from build123d import *

# Parameters (mm, degrees)
SKETCH1_R           = 76.2
BOSS_EXTRUDE1_DEPTH = 130
SKETCH1_3_R         = 72.2
CUT_EXTRUDE1_DEPTH  = 126
FILLET1_R           = 5


with BuildPart() as part:
    # Sketch1 → Boss-Extrude1 (new body)
    with BuildSketch(Plane(origin=(0, 0, 0), x_dir=(1, 0, 0), z_dir=(0, 1, 0))):
        with Locations(Location((0, 0, 0), (0, 0, 270))):
            Circle(SKETCH1_R)
        with BuildLine():
            Line((-3.175, -5), (-3.175, 5))
            ThreePointArc((-3.175, 5), (0, 8.175), (3.175, 5))
            Line((3.175, 5), (3.175, -5))
            ThreePointArc((3.175, -5), (0, -8.175), (-3.175, -5))
        make_face(mode=Mode.SUBTRACT)
    extrude(amount=BOSS_EXTRUDE1_DEPTH)

    # Sketch1<3> → Cut-Extrude1 (cut)
    with BuildSketch(Plane(origin=(0, 0, 0), x_dir=(1, 0, 0), z_dir=(0, 1, 0))):
        with Locations(Location((0, 0, 0), (0, 0, 270))):
            Circle(SKETCH1_3_R)
    extrude(amount=CUT_EXTRUDE1_DEPTH, mode=Mode.SUBTRACT)

    # Fillet1
    fillet1_edges = [part.edges().sort_by_distance(p)[0] for p in [
        (0, 130, -76.2),
    ]]
    fillet(fillet1_edges, radius=FILLET1_R)


solid = part.part
The model under review builds one solid part; all positions refer to its coordinate system, in mm. A direction names the side the tool comes from. Give positions to 0.01 mm unless a question says otherwise; leave off trailing zeros. Write each loop counter-clockwise with the first axis right and the second up, starting at its lowest first coordinate (ties: lowest second). Pieces come first, ordered by that corner, then holes.
1. For P1, Ø6, axis at x = 23, z = -51.5, coming from the -Y side; P2, Ø10, axis at y = 16.5, z = -9, coming from the -X side; P3, Ø8, axis at y = 60.5, z = 44.5, coming from the -X side, all flat-tipped, find the tip position at first contact; note any pin that passes through.
2. Tool access review of faces 1 (the flat face through (-15, 130, -1)), 2 (the flat face through (-3.175, 128, 0)), 3 (the cylindrical face through (-43.933, 62.118, -57.295)): name each direction out of +Z, -Z, +X, -X, +Y, -Y from which nothing blocks a thin tool from reaching the whole face with its end or side.
3. Add section B-B, the plane x = 0. Write out the cut boundary in (y, z) (3 decimals), plus the area to 3 significant figures.
4. Wall thickness on L1, parallel to X at y = 67, z = 0; L2, parallel to Z at x = 21.5, y = 71.5; L3, parallel to Y at x = 25, z = -61.5: over which ranges is each line inside the solid? List them lowest first.
5. Add section C-C, the plane y = 27.5. Write out the cut boundary in (x, z).
6. Draft analysis for pull direction X (two halves, no side actions). For faces 4 (the cylindrical face through (-46.367, 61.625, -60.47)), 5 (the flat face through (46, 0, 56)), 6 (the cylindrical face through (-0.07, 127.972, -8.174)), state which applies: +X half, -X half, draft (parallel to the pull), parting line (faces both ways), or undercut.
7. Add section A-A, the plane z = 0. Write out the cut boundary in (x, y) (3 decimals).
Worked answers:
1. P1: stops at y = 126
1. P2: stops at x = -76.09
1. P3: stops at x = -64.55
2. face 1: +Z, -Z, +X, -X, +Y
2. face 2: +Y, -Y
2. face 3: -Y
3. outline: (0, -76.2) - (125, -76.2) arc R5 ccw to (130, -71.2) - (130, -8.175) - (126, -8.175) - (126, -72.2) - (0, -72.2) - close; (0, 72.2) - (126, 72.2) - (126, 8.175) - (130, 8.175) - (130, 71.2) arc R5 ccw to (125, 76.2) - (0, 76.2) - close
3. area: 1,540 mm2
4. L1: x = -76.2 to -72.2, 72.2 to 76.2
4. L2: z = -73.1 to -68.92, 68.92 to 73.1
4. L3: y = 126 to 130
5. outline: circle Ø152.4 at (0, 0); hole circle Ø144.4 at (0, 0)
6. face 4: parting line
6. face 5: draft
6. face 6: undercut
7. outline: (-76.2, 0) - (-72.2, 0) - (-72.2, 126) - (-3.175, 126) - (-3.175, 130) - (-71.2, 130) arc R5 ccw to (-76.2, 125) - close; (3.175, 126) - (72.2, 126) - (72.2, 0) - (76.2, 0) - (76.2, 125) arc R5 ccw to (71.2, 130) - (3.175, 130) - close
